Here's how the part is built. I have some questions about the finished solid (model axes, mm). A direction names the side the tool comes from. Coordinates: 2 decimals unless noted, no trailing zeros. Write each loop counter-clockwise with the first axis right and the second up, starting at its lowest first coordinate (ties: lowest second). Pieces come first, ordered by that corner, then holes.
Item 1: I want a section at B-B (x = 394.5). Please give me the cut outline in (y, z), and give its area (3 significant figures).
Item 2: Please list where these lines run through material, in increasing order: line 1 (Y direction, x = 253, z = -3.8); line 2 (Z direction, x = 239, y = -3); line 3 (X direction, y = -0.75, z = -0.75).
Item 3: I'm going to push flat-ended pins straight in: P1, Ø2.5, axis at x = 253, y = -4.5, coming from the -Z side; P2, Ø2, axis at x = 119.5, y = -3.5, coming from the +Z side. Where does each tip first touch, or does it pass through?
Item 4: I want a section at A-A (y = -4.5). Please give me the cut outline in (x, z).
Item 5: For faces 1 (the face through (215, -5, -3.5)), 2 (the face through (215, 0, 0)), which set-ups out of +Z, -Z, +X, -X, +Y, -Y let a thin tool reach every point of the face, with its end or its side?
from build123d import *

# Parameters (mm, degrees)
PAD017_DEPTH      = 440
PAD017_DEPTH_BACK = 16
POCKET018_DEPTH   = 5
SKETCH055_R       = 1.5
POCKET019_DEPTH   = 5


with BuildPart() as part:
    # Sketch053 → Pad017 (new body, two sides)
    with BuildSketch(Plane.YZ) as pad017_sk:
        Polygon((0, -4.5), (-8, -4.5), (-8, -3.5), (-1, -3.5), (-1, 3.5), (0, 3.5), align=None)
    extrude(amount=PAD017_DEPTH)
    extrude(pad017_sk.sketch, amount=-PAD017_DEPTH_BACK)

    # Sketch054 → Pocket018 (cut)
    with BuildSketch(Plane.XZ):
        with BuildLine():
            ThreePointArc((-6, 1.6), (-7.6, 0), (-6, -1.6))
            Line((-6, -1.6), (0, -1.6))
            ThreePointArc((0, -1.6), (1.6, 0), (0, 1.6))
            Line((0, 1.6), (-6, 1.6))
        make_face()
        with BuildLine():
            Line((-16.5, 4), (-10.5, 4))
            Line((-10.5, 4), (-11.4360006338, -0.3374996039))
            ThreePointArc((-14.6, 0), (-13.1697071214, -1.5909743848), (-11.4360006338, -0.3374996039))
            Line((-14.6, 0), (-14.6, 1.25))
            ThreePointArc((-14.6, 1.25), (-14.7801442911, 1.6343075923), (-15.1907693019, 1.7416919095))
            Line((-15.1907693019, 1.7416919095), (-16.5, 1.5))
            Line((-16.5, 1.5), (-16.5, 4))
        make_face()
    extrude(amount=POCKET018_DEPTH, mode=Mode.SUBTRACT)

    # Sketch055 → Pocket019 (cut)
    with BuildSketch(Plane.XY):
        with Locations((425, -4.5)):
            Circle(SKETCH055_R)
        with Locations((253, -4.5)):
            Circle(SKETCH055_R)
    extrude(amount=-POCKET019_DEPTH, mode=Mode.SUBTRACT)


solid = part.part
Answer:
1. outline: (-8, -4.5) - (0, -4.5) - (0, 3.5) - (-1, 3.5) - (-1, -3.5) - (-8, -3.5) - close
1. area: 15.0 mm2
2. line 1: y = -8 to -6, -3 to 0
2. line 2: z = -4.5 to -3.5
2. line 3: x = -16 to -14.41, -11.59 to -7.41, 1.41 to 440
3. P1: passes through
3. P2: stops at z = -3.5
4. outline: (-16, -4.5) - (251.5, -4.5) - (251.5, -3.5) - (-16, -3.5) - close; (254.5, -4.5) - (423.5, -4.5) - (423.5, -3.5) - (254.5, -3.5) - close; (426.5, -4.5) - (440, -4.5) - (440, -3.5) - (426.5, -3.5) - close
5. face 1: +Z, +X, -X, -Y
5. face 2: +Z, -Z, +X, -X, +Y
